Work out the finished part from the listing and answer in its coordinate system (mm). A direction names the side the tool comes from. Coordinates: 2 decimals unless noted, no trailing zeros. Loops run counter-clockwise (first coordinate to the right, second up) from the corner with the lowest first, then second, coordinate; pieces in that order, holes last.
```python
from build123d import *

# Parameters (mm, degrees)
F1_DEPTH = 6.35
F2_SCALE = 0.5


with BuildPart() as f1:
    # F0 (on Front) → F1 (new body, symmetric)
    with BuildSketch(Plane.XZ):
        with BuildLine():
            ThreePointArc((-11.5290090528, -23.8732525036), (-9.8294039198, -25.6783091317), (-7.850968465, -27.1725247086))
            Line((-7.850968465, -27.1725247086), (-7.850968465, -14.7204540884))
            Line((-7.850968465, -14.7204540884), (-7.850968465, -7.9911025987))
            Line((-7.850968465, -7.9911025987), (-11.5290090528, -7.9911025987))
            Line((-11.5290090528, -7.9911025987), (-11.5290090528, -23.8732525036))
        make_face()
        with BuildLine():
            Line((-7.850968465, -30.5458810074), (-7.850968465, -27.1725247086))
            ThreePointArc((-7.850968465, -27.1725247086), (-9.8294039198, -25.6783091317), (-11.5290090528, -23.8732525036))
            Line((-11.5290090528, -23.8732525036), (-11.5290090528, -30.5458810074))
            Line((-11.5290090528, -30.5458810074), (-7.850968465, -30.5458810074))
        make_face()
        Polygon((5.1503910808, 19.6066750714), (5.1503910808, 11.4153277746), (5.1503910808, 6.3087673495), (8.0611995911, 6.3087673495), (8.0611995911, 24.3938967455), (5.1503910808, 24.3938967455), (5.1503910808, 22.4311687176), align=None)
        with BuildLine():
            ThreePointArc((-5.8608669981, -28.2238613102), (14.4129812082, -17.7134026782), (0, 0))
            ThreePointArc((0, 0), (-6.2617137528, 9.6947188107), (5.1503910808, 11.4153277746))
            Line((5.1503910808, 11.4153277746), (5.1503910808, 19.6066750714))
            ThreePointArc((5.1503910808, 19.6066750714), (4.1758661078, 19.9585920865), (3.1775916397, 20.236067482))
            ThreePointArc((3.1775916397, 20.236067482), (2.4268766545, 20.2483751203), (1.7196691769, 20.5005299348))
            ThreePointArc((1.7196691769, 20.5005299348), (-13.7119930511, 7.7310759956), (0, -6.8694856234))
            ThreePointArc((0, -6.8694856234), (5.5514730405, -20.2719271289), (-7.850968465, -14.7204540884))
            Line((-7.850968465, -14.7204540884), (-7.850968465, -27.1725247086))
            ThreePointArc((-7.850968465, -27.1725247086), (-6.8760406561, -27.7362841988), (-5.8608669981, -28.2238613102))
        make_face()
        with BuildLine():
            ThreePointArc((1.7196691769, 20.5005299348), (2.4268766545, 20.2483751203), (3.1775916397, 20.236067482))
            ThreePointArc((3.1775916397, 20.236067482), (2.4521981922, 20.3879671044), (1.7196691769, 20.5005299348))
        make_face()
        with BuildLine():
            ThreePointArc((3.1775916397, 20.236067482), (4.1758661078, 19.9585920865), (5.1503910808, 19.6066750714))
            Line((5.1503910808, 19.6066750714), (5.1503910808, 22.4311687176))
            ThreePointArc((5.1503910808, 22.4311687176), (4.5596761112, 20.9780050452), (3.1775916397, 20.236067482))
        make_face()
        with BuildLine():
            ThreePointArc((-7.850968465, -30.5458810074), (-7.2853702731, -29.0168061791), (-5.8608669981, -28.2238613102))
            ThreePointArc((-5.8608669981, -28.2238613102), (-6.8760406561, -27.7362841988), (-7.850968465, -27.1725247086))
            Line((-7.850968465, -27.1725247086), (-7.850968465, -30.5458810074))
        make_face()
    extrude(amount=F1_DEPTH, both=True)


with BuildPart() as f1_1:
    # F2: moved
    add(f1.part.scale(F2_SCALE))


solid = f1_1.part
```
1. Determine the mould class of faces 1 (the flat face through (-5.765, 0, -10)), 2 (the flat face through (-5, 0, -15.273)), 3 (the cylindrical face through (-3.17, -0.04, 4.76)) for opening direction X: released by +X, released by -X, zero draft, split by the parting line, or undercut.
2. Each of these flat-tipped pins is pushed along its axis until it touches: P1, Ø0.7, axis at x = 3.5, y = 0.5, coming from the -Z side; P2, Ø3, axis at x = 4, y = -1, coming from the -Z side; P3, Ø0.8, axis at y = 0, z = 4, coming from the -X side. Where does it stop, or does it pass through?
3. A cutting plane is placed at C-C, the plane y = -0.75. Give the vertices of the cut face in (x, z), then the cut area to 3 significant figures.
4. A cutting plane is placed at A-A, the plane x = 0. Give the vertices of the cut face in (y, z) (3 decimals).
5. For faces 4 (the cylindrical face through (-3.65, -0.04, -14.52)), 5 (the flat face through (2.575, 0, 4)), 6 (the cylindrical face through (2.29, -0.04, 10.5)), 7 (the flat face through (2.575, 0, 12)), 8 (the flat face through (4.031, 0, 8)), determine the directions among +Z, -Z, +X, -X, +Y, -Y from which every point of the face is accessible in a straight line to the end or side of a thin tool.
6. A cutting plane is placed at B-B, the plane z = -8.5. Give the vertices of the cut face in (x, y) (1 decimal).
7. Straight lines are drawn through the part: probe 1 along X at (y, z) = (1.5, -7.5); probe 2 along Z at (x, y) = (-1.5, 1.5); probe 3 along Z at (x, y) = (-1.75, 1.5). For each, find the intervals that lie inside material, in ascending order.
8. A cutting plane is placed at D-D, the plane z = -2.75. Give the vertices of the cut face in (x, y) (3 decimals).
Answers below:
1. face 1: released by -X
1. face 2: zero draft
1. face 3: undercut
2. P1: stops at z = -14.01
2. P2: stops at z = -14.28
2. P3: stops at x = -6.87
3. outline: (-5.76, -15.27) - (-3.93, -15.27) arc R1.17 cw to (-2.93, -14.11) arc R7.36 ccw (long way) to (0, 0) arc R3.43 cw (long way) to (2.58, 5.71) - (2.58, 3.15) - (4.03, 3.15) - (4.03, 12.2) - (2.58, 12.2) - (2.58, 11.22) arc R1.16 cw to (1.59, 10.12) arc R6.87 ccw (long way) to (0, -3.43) arc R3.93 cw (long way) to (-3.93, -7.36) - (-3.93, -4) - (-5.76, -4) - close
3. area: 176 mm2
4. outline: (-3.175, -14.72) - (3.175, -14.72) - (3.175, -11.286) - (-3.175, -11.286) - close; (-3.175, -3.435) - (3.175, -3.435) - (3.175, 0) - (-3.175, 0) - close; (-3.175, 6.87) - (3.175, 6.87) - (3.175, 10.304) - (-3.175, 10.304) - close
5. face 4: -Z, +Y, -Y
5. face 5: +Y, -Y
5. face 6: +Z, +Y, -Y
5. face 7: +Z, -X, +Y, -Y
5. face 8: +Z, +X, +Y, -Y
6. outline: (-5.8, -3.2) - (-3.8, -3.2) - (-3.8, 3.2) - (-5.8, 3.2) - close; (3.8, -3.2) - (7.3, -3.2) - (7.3, 3.2) - (3.8, 3.2) - close
7. probe 1: x = -5.76 to -3.92, 3.92 to 7.36
7. probe 2: z = -14.57 to -10.99, -3.27 to 0.34, 6.52 to 10.14
7. probe 3: z = -14.51 to -10.87, -3.21 to 0.48, 6.39 to 10.08
8. outline: (-2.99, -3.175) - (5.737, -3.175) - (5.737, 3.175) - (-2.99, 3.175) - close
